The figure shows three views and two pictorial views of one solid part (mm, origin at its lowest corner). Answer the questions. A direction names the side the tool comes from. Coordinates: 2 decimals unless noted, no trailing zeros. Loops run counter-clockwise (first coordinate to the right, second up) from the corner with the lowest first, then second, coordinate; pieces in that order, holes last. Notation, with made-up numbers: (16, 8.25) -> (32, 8.25) arc R12 cw to (32, 15.25) -> close; hole circle Ø7 at (78.5, 7.5). An arc over 180 degrees is marked (long way). Answer as a JSON object with one key per item and string values. Group by question number.
1) Section C-C, the plane z = 4.5 is taken. Give the vertices of the cut face in (x, y) (1 decimal).
2) Flat-ended cylindrical pins translate along their axes: P1, Ø1.5, axis at y = 6.5, z = 3.5, coming from the -X side; P2, Ø1.5, axis at x = 4.325, y = 10.675, coming from the -Z side; P3, Ø3, axis at y = 11, z = 13.5, coming from the -X side; P4, Ø8, axis at y = 1.5, z = 10, coming from the +X side. Find the tip coordinate at first contact, or state that the pin passes through.
3) Section A-A, the plane x = 7.5 is taken. Give the vertices of the cut face in (y, z) (3 decimals), plus the area to 3 significant figures.
4) Section D-D, the plane x = 12 is taken. Give the vertices of the cut face in (y, z), plus the area to 3 significant figures.
5) Which of the six approach directions +Z, -Z, +X, -X, +Y, -Y give full straight-line access (tool end or side, diameter ignored) to the marked faces 1 and 2?
6) Consider probe 1 along Y at (x, z) = (3.75, 2.25); probe 2 along X at (y, z) = (11, 17). Determine where each line is inside the solid, lowest interval first. Write a range as [from, to].
7) Determine the mould class of the marked faces 3, 4 and 5 for opening direction Y: released by +Y, released by -Y, zero draft, split by the parting line, or undercut.
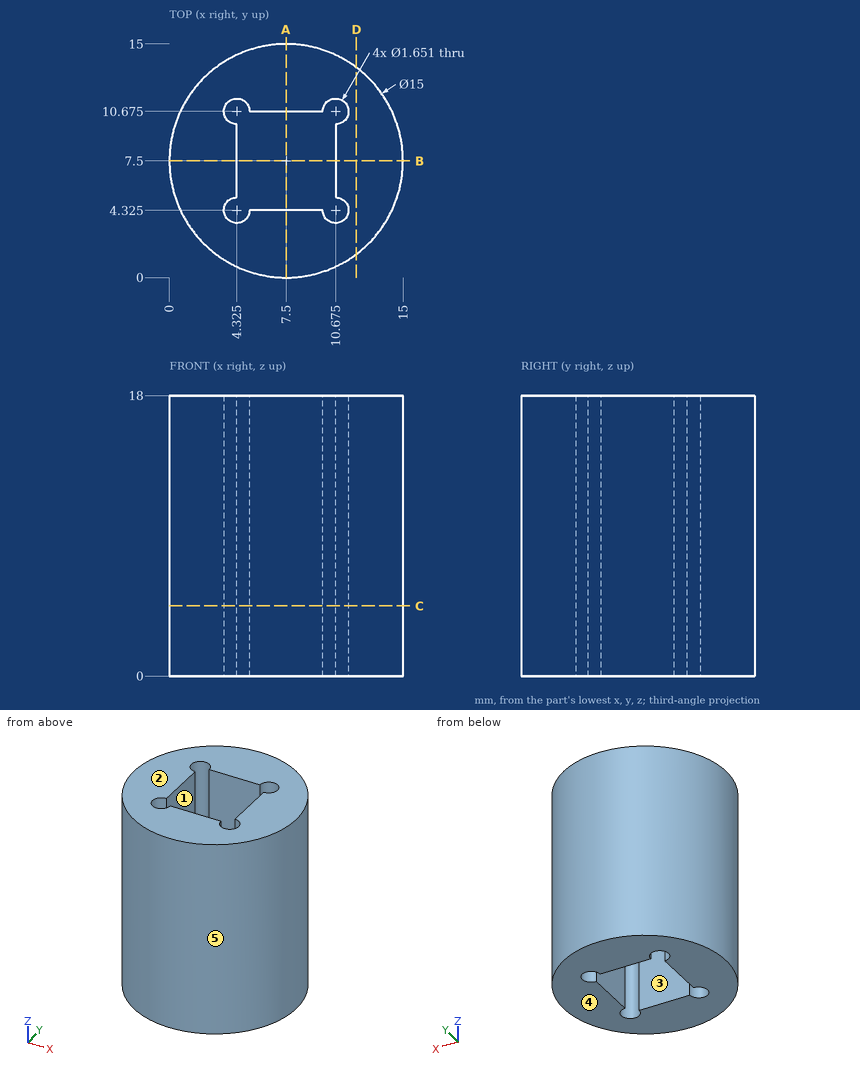
Determined:
{
 "1": {"outline": "circle Ø15 at (7.5, 7.5); hole (4.3, 5.2) arc R0.8 ccw (long way) to (5.2, 4.3) -> (9.8, 4.3) arc R0.8 ccw (long way) to (10.7, 5.2) -> (10.7, 9.8) arc R0.8 ccw (long way) to (9.8, 10.7) -> (5.2, 10.7) arc R0.8 ccw (long way) to (4.3, 9.8) -> close"},
 "2": {"P1": "x = 0", "P2": "through", "P3": "x = 0.27", "P4": "x = 14.73"},
 "3": {"outline": "(0, 0) -> (4.325, 0) -> (4.325, 18) -> (0, 18) -> close; (10.675, 0) -> (15, 0) -> (15, 18) -> (10.675, 18) -> close", "area": "156 mm²"},
 "4": {"outline": "(1.5, 0) -> (13.5, 0) -> (13.5, 18) -> (1.5, 18) -> close", "area": "216 mm²"},
 "5": {"face 1": "+Z, -Z", "face 2": "+Z, +X, -X, +Y, -Y"},
 "6": {"probe 1": "[1, 3.73], [4.92, 10.08], [11.27, 14]", "probe 2": "[0.87, 3.57], [5.08, 9.92], [11.43, 14.13]"},
 "7": {"face 3": "undercut", "face 4": "zero draft", "face 5": "split by the parting line"}
}
